Design review of the part built by this model. Coordinates are the model's own, in mm. A direction names the side the tool comes from. Give positions to 0.01 mm unless a question says otherwise; leave off trailing zeros. Order: outer loops, then holes, each group sorted by start corner. A loop starts at its lowest first (then second) coordinate and runs counter-clockwise, first axis right, second up.
```python
from build123d import *

# Parameters (mm, degrees)
F0_W      = 32
F0_H      = 40
F0_R      = 11.1
F0_R_2    = 5.175
F1_DEPTH  = 10
F0_R_3    = 2.675
F2_DEPTH  = 5
F3_DEPTH  = 5
F4_SIZE   = 0.5
F5_DEPTH  = 10
F6_DEPTH  = 10
F8_SIZE   = 2
F0_R_4    = 9.1
F9_DEPTH  = 10
F10_DEPTH = 8.5
F11_R     = 15
F12_SIZE  = 0.49999


# Not quite as in the source:
# - a fillet or chamfer is up to 0.001 mm smaller than in the source, because OpenCascade refuses the exact size
# - a feature of the source that left no trace in its solid (it failed there, or was rolled back) is left out


with BuildPart() as f1:
    # F0 (on Top) → F1 (new body)
    with BuildSketch(Plane.XY):
        with Locations((-1.076085493, 10.825)):
            Rectangle(F0_W, F0_H)
        with Locations((-1.076085493, 13.645)):
            Circle(F0_R, mode=Mode.SUBTRACT)
        Polygon((14.923914507, -9.175), (-17.076085493, -9.175), (-27.076085493, -9.175), (-27.076085493, -29.175), (-17.076085493, -29.175), (14.923914507, -29.175), (24.923914507, -29.175), (24.923914507, -9.175), align=None)
        with Locations((-19.901085493, -19.175)):
            Circle(F0_R_2, mode=Mode.SUBTRACT)
        with Locations((17.748914507, -19.175)):
            Circle(F0_R_2, mode=Mode.SUBTRACT)
    extrude(amount=F1_DEPTH)

    # F0 (on Top) → F2 (join)
    with BuildSketch(Plane.XY):
        with Locations((-19.901085493, -19.175)):
            Circle(F0_R_2)
        with Locations((-19.901085493, -19.175)):
            Circle(F0_R_3, mode=Mode.SUBTRACT)
    extrude(amount=F2_DEPTH)

    # F0 (on Top) → F3 (join)
    with BuildSketch(Plane.XY):
        with Locations((17.748914507, -19.175)):
            Circle(F0_R_2)
        with Locations((17.748914507, -19.175)):
            Circle(F0_R_3, mode=Mode.SUBTRACT)
    extrude(amount=F3_DEPTH)

    # F4
    f4_edges = [f1.edges().sort_by_distance(p)[0] for p in [
        (-27.076085, -19.175, 10),
        (-22.076085, -9.175, 10),
        (19.923915, -9.175, 10),
        (24.923915, -19.175, 10),
        (24.923915, -9.175, 5),
        (-27.076085, -9.175, 5),
        (-27.076085, -29.175, 5),
        (24.923915, -29.175, 5),
        (-1.076085, -29.175, 10),
        (-17.076085, 10.825, 10),
        (14.923915, 10.825, 10),
    ]]
    chamfer(f4_edges, length=F4_SIZE)

    # F0 (on Top) → F5 (join)
    with BuildSketch(Plane.XY):
        Polygon((14.923914507, -9.175), (-17.076085493, -9.175), (-27.076085493, -9.175), (-27.076085493, -29.175), (-17.076085493, -29.175), (14.923914507, -29.175), (24.923914507, -29.175), (24.923914507, -9.175), align=None)
        with Locations((-19.901085493, -19.175)):
            Circle(F0_R_2, mode=Mode.SUBTRACT)
        with Locations((17.748914507, -19.175)):
            Circle(F0_R_2, mode=Mode.SUBTRACT)
    extrude(amount=-F5_DEPTH)

    # F0 (on Top) → F6 (join)
    with BuildSketch(Plane.XY):
        with Locations((17.748914507, -19.175)):
            Circle(F0_R_2)
        with Locations((17.748914507, -19.175)):
            Circle(F0_R_3, mode=Mode.SUBTRACT)
        with Locations((-19.901085493, -19.175)):
            Circle(F0_R_2)
        with Locations((-19.901085493, -19.175)):
            Circle(F0_R_3, mode=Mode.SUBTRACT)
    extrude(amount=-F6_DEPTH)

    # F8
    f8_edges = [f1.edges().sort_by_distance(p)[0] for p in [
        (-1.076085, -9.175, -10),
    ]]
    chamfer(f8_edges, length=F8_SIZE)

    # F0 (on Top) → F9 (join)
    with BuildSketch(Plane.XY):
        with Locations((-1.076085493, 13.645)):
            Circle(F0_R)
        with Locations((-1.076085493, 13.645)):
            Circle(F0_R_4, mode=Mode.SUBTRACT)
    extrude(amount=F9_DEPTH)

    # F0 (on Top) → F10 (cut)
    with BuildSketch(Plane.XY):
        with Locations((-1.076085493, 13.645)):
            Circle(F0_R)
        with Locations((-1.076085493, 13.645)):
            Circle(F0_R_4, mode=Mode.SUBTRACT)
    extrude(amount=F10_DEPTH, mode=Mode.SUBTRACT)

    # F11
    f11_edges = [f1.edges().sort_by_distance(p)[0] for p in [
        (14.923915, 30.825, 4.75),
        (-17.076085, 30.825, 4.75),
    ]]
    fillet(f11_edges, radius=F11_R)

    # F12 (size 0.5 in the source; OpenCascade refuses exactly that, so slightly less here)
    f12_edges = [f1.edges().sort_by_distance(p)[0] for p in [
        (10.530516, 26.431602, 0),
        (-11.224621, 27.712148, 10),
        (9.07245, 27.712148, 10),
        (-1.076085, 30.825, 10),
        (-1.076085, 30.825, 0),
        (-12.682687, 26.431602, 0),
        (-17.076085, 3.325, 0),
        (-27.076085, -9.175, -4),
        (24.923915, -9.175, -4),
        (14.923915, 3.325, 0),
        (-27.076085, -29.175, -5),
        (24.923915, -29.175, -5),
    ]]
    chamfer(f12_edges, length=F12_SIZE)


solid = f1.part
```
1. Take a section at A-A (y = -7.5). State the section outline as (x, z) points.
Recorded:
outline: (-17.08, 0.5) - (-16.58, 0) - (14.42, 0) - (14.92, 0.5) - (14.92, 9.5) - (14.42, 10) - (-16.58, 10) - (-17.08, 9.5) - close
2. For line 1 along X through (y, z) = (-20.5, -3); line 2 along Y through (x, z) = (13, -2.5) (3 decimals); line 3 along Z through (x, y) = (-2, -0.5), list the stretches that pass through material, from the lowest coordinate up.
Recorded:
line 1: x = -27.08 to -22.22, -17.58 to 15.43, 20.07 to 24.92
line 2: y = -29.175 to -9.175
line 3: z = 0 to 10
3. Machinability: for faces 1 (the face through (14.924, 3, 5)), 2 (the face through (20, -21, 5)), 3 (the face through (-17.076, 3, 5)), which of the approach directions +Z, -Z, +X, -X, +Y, -Y give a long, thin tool a straight path to every point of the face, cutting with its end or side? Answer none if there is none.
Recorded:
face 1: +Z, -Z, +X, +Y
face 2: +Z
face 3: +Z, -Z, -X, +Y
4. Draft analysis for pull direction Y (two halves, no side actions). For faces 4 (the face through (-1, -29.175, 0)), 5 (the face through (10.41, 26.55, 5.06)), 6 (the face through (-8.3, 8.11, 9.24)), state which applies: pulls with the +Y half, pulls with the -Y half, needs draft (parallel to the pull), parting line crosses it, or undercut.
Recorded:
face 4: pulls with the -Y half
face 5: pulls with the +Y half
face 6: undercut
5. Take a section at C-C (z = 3.75). State the section outline as (x, y) points (3 decimals).
Recorded:
outline: (-27.076, -28.675) - (-26.576, -29.175) - (24.424, -29.175) - (24.924, -28.675) - (24.924, -9.675) - (24.424, -9.175) - (14.924, -9.175) - (14.924, 15.825) arc R15 ccw to (-0.076, 30.825) - (-2.076, 30.825) arc R15 ccw to (-17.076, 15.825) - (-17.076, -9.175) - (-26.576, -9.175) - (-27.076, -9.675) - close; hole circle Ø5.35 at (-19.901, -19.175); hole circle Ø22.2 at (-1.076, 13.645); hole circle Ø5.35 at (17.749, -19.175)
6. Take a section at D-D (y = 12.5). State the section outline as (x, z) points, then the cut area to 3 significant figures.
Recorded:
outline: (-17.08, 0.5) - (-16.58, 0) - (-12.12, 0) - (-12.12, 8.5) - (-10.1, 8.5) - (-10.1, 10) - (-16.58, 10) - (-17.08, 9.5) - close; (7.95, 8.5) - (9.96, 8.5) - (9.96, 0) - (14.42, 0) - (14.92, 0.5) - (14.92, 9.5) - (14.42, 10) - (7.95, 10) - close
area: 105 mm2
7. Take a section at B-B (x = 16.5). State the section outline as (y, z) points (3 decimals), then the cut area to 3 significant figures.
Recorded:
outline: (-29.175, -10) - (-21.541, -10) - (-21.541, 5) - (-24.197, 5) - (-24.197, 10) - (-28.675, 10) - (-29.175, 9.5) - close; (-16.809, -10) - (-11.175, -10) - (-9.175, -8) - (-9.175, 9.5) - (-9.675, 10) - (-14.153, 10) - (-14.153, 5) - (-16.809, 5) - close
area: 277 mm2
8. For pin 1 (5 mm diameter, centred on x = 16.5, y = -17.5, fed in from +Z); pin 2 (4.5 mm diameter, centred on y = -1.5, z = 5, fed in from +X); pin 3 (1.5 mm diameter, centred on y = 19.5, z = 3.5, fed in from -X), all flat-tipped, find the tip position at first contact; note any pin that passes through.
Recorded:
pin 1: stops at z = 5
pin 2: stops at x = 14.92
pin 3: stops at x = -16.79
